For this review, use the dimensioned drawing (mm, ordinates from the lowest corner) and the shaded views. Coordinates: 2 decimals unless noted, no trailing zeros. Order: outer loops, then holes, each group sorted by start corner. A loop starts at its lowest first (then second) coordinate and runs counter-clockwise, first axis right, second up. Notation, with made-up numbers: M 3.5,50.25 L 30.5,50.25 A17 cw 30.5,60.25 Z; hole C 47,60.25 d9. An arc over 180 degrees is marked long. Answer in a Markdown table with one row per item.
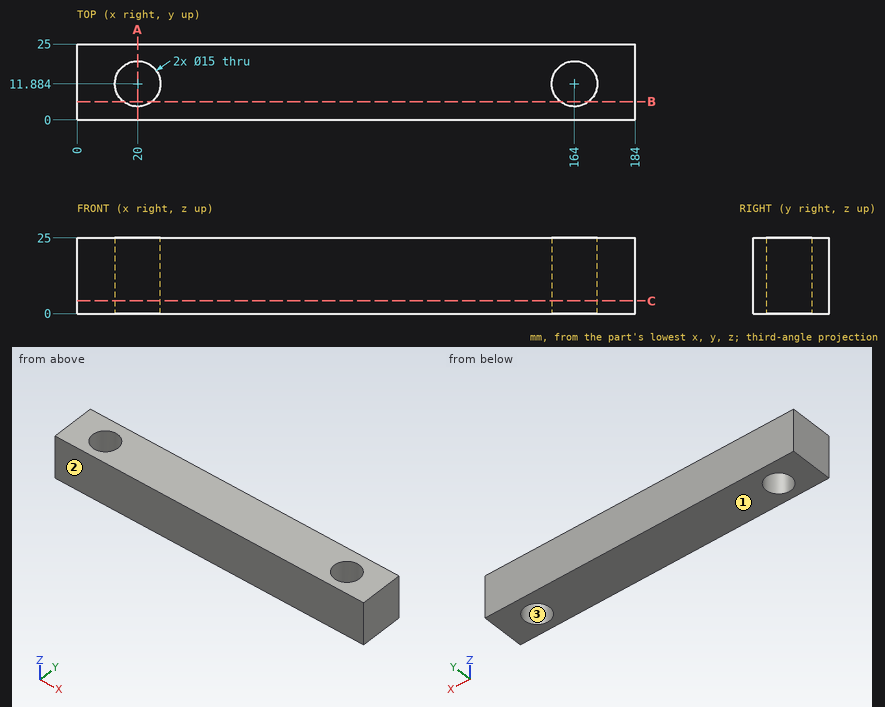
(1) For line 1 along X through (y, z) = (5.75, 12.25) (1 decimal); line 2 along X through (y, z) = (8.25, 2.5); line 3 along Y through (x, z) = (20, 8.25), list the stretches that pass through material, from the lowest coordinate up. Write a range as from..to.
Return value:
| item | result |
|---|---|
| line 1 | x = 0..15.7, 24.3..159.7, 168.3..184 |
| line 2 | x = 0..13.44, 26.56..157.44, 170.56..184 |
| line 3 | y = 0..4.38, 19.38..25 |
(2) Add section C-C, the plane z = 4.25. Give the boundary of the cut face in (x, y).
Return value:
| item | result |
|---|---|
| outline | M 0,0 L 184,0 L 184,25 L 0,25 Z; hole C 20,11.88 d15; hole C 164,11.88 d15 |
(3) Add section A-A, the plane x = 20. Give the boundary of the cut face in (y, z).
Return value:
| item | result |
|---|---|
| outline | M 0,0 L 4.38,0 L 4.38,25 L 0,25 Z; M 19.38,0 L 25,0 L 25,25 L 19.38,25 Z |
(4) Add section B-B, the plane y = 6. Give the boundary of the cut face in (x, z).
Return value:
| item | result |
|---|---|
| outline | M 0,0 L 15.35,0 L 15.35,25 L 0,25 Z; M 24.65,0 L 159.35,0 L 159.35,25 L 24.65,25 Z; M 168.65,0 L 184,0 L 184,25 L 168.65,25 Z |
(5) Insertion check: pin 1 Ø10 at (y, z) = (17.5, 14) entering from -X. The pin has a flat end and moves straight along its axis. Give the tip position at first contact, or say it passes through.
Return value:
| item | result |
|---|---|
| pin 1 | stops at x = 0 |
(6) Draft analysis for pull direction Y (two halves, no side actions). For the marked faces 1, 2 and 3, state which applies: pulls with the +Y half, pulls with the -Y half, needs draft (parallel to the pull), parting line crosses it, or undercut.
Return value:
| item | result |
|---|---|
| face 1 | needs draft |
| face 2 | pulls with the -Y half |
| face 3 | undercut |
